Build history of the part. All positions in model axes, mm. Face numbers are marked on the shaded views. A direction names the side the tool comes from. Round coordinates to 2 decimals unless told otherwise and drop trailing zeros. Loops run counter-clockwise (first coordinate to the right, second up) from the corner with the lowest first, then second, coordinate; pieces in that order, holes last.
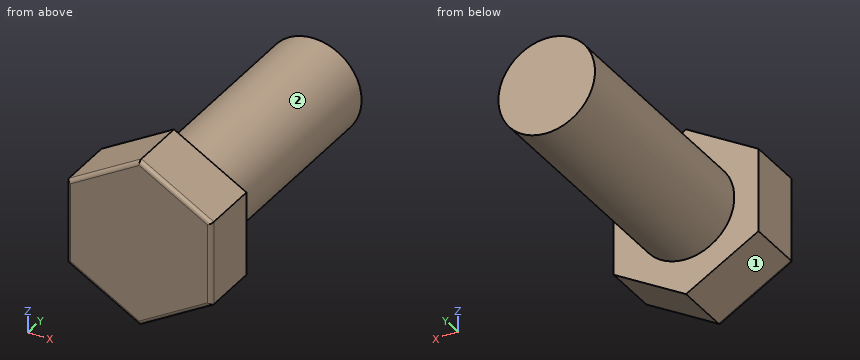
from build123d import *

# Parameters (mm, degrees)
EXTRUDE_1_DEPTH = 15
SKETCH_2_R      = 12
EXTRUDE_2_DEPTH = 60
FILLET_1_R      = 1


with BuildPart() as part:
    # 草圖1 → 填料-伸長1 (new body)
    with BuildSketch(Plane(origin=(0, 0, 0), x_dir=(1, 0, 0), z_dir=(0, 1, 0))):
        Polygon((18, -10.392304845), (18, 10.392304845), (0, 20.784609691), (-18, 10.392304845), (-18, -10.392304845), (0, -20.784609691), align=None)
    extrude(amount=EXTRUDE_1_DEPTH)

    # 草圖2 → 填料-伸長2 (add)
    with BuildSketch(Plane(origin=(0, 15, 0), x_dir=(1, 0, 0), z_dir=(0, 1, 0))):
        Circle(SKETCH_2_R)
    extrude(amount=EXTRUDE_2_DEPTH)

    # 圓角1
    fillet_1_edges = [part.edges().sort_by_distance(p)[0] for p in [
        (18, 0, 0),
        (9, 0, 15.588457268),
        (-9, 0, 15.588457268),
        (-18, 0, 0),
        (-9, 0, -15.588457268),
        (9, 0, -15.588457268),
    ]]
    fillet(fillet_1_edges, radius=FILLET_1_R)


solid = part.part
(1) Pin check, flat tips, straight feed: P1, Ø1, axis at x = 8.5, z = -16, coming from the -Y side; P2, Ø2, axis at y = 30.5, z = -3, coming from the +X side; P3, Ø1, axis at x = 3, y = 10, coming from the +Z side; P4, Ø8, axis at x = -12.5, z = 7, coming from the +Y side. Stop position of each tip, or through.
Responses:
P1: stops at y = 0.2
P2: stops at x = 11.83
P3: stops at z = 19.34
P4: stops at y = 75
(2) Slice it at C-C on z = -7.5. List the corners of the cut face in (x, y).
Responses:
outline: (-18, 1) arc R1 ccw to (-17, 0) - (17, 0) arc R1 ccw to (18, 1) - (18, 15) - (9.37, 15) - (9.37, 75) - (-9.37, 75) - (-9.37, 15) - (-18, 15) - close
(3) Which spindle directions (+Z, -Z, +X, -X, +Y, -Y) get a long thin tool onto all of the face, cutting with end or side? Do the marked faces 1 and 2. Say none if no direction does.
Responses:
face 1: -Z, -X, +Y, -Y
face 2: +Y
(4) Probe line 1 (Y direction, x = -11, z = 9); line 2 (X direction, y = 56, z = -6.5); line 3 (X direction, y = 19.5, z = -11). List the from-to ranges inside material, lowest first.
Responses:
line 1: y = 0 to 15
line 2: x = -10.09 to 10.09
line 3: x = -4.8 to 4.8
(5) Slice it at D-D on y = 66. List the corners of the cut face in (x, z), plus the area to 3 significant figures.
Responses:
outline: circle Ø24 at (0, 0)
area: 452 mm2
(6) Slice it at B-B on z = 0. List the corners of the cut face in (x, y).
Responses:
outline: (-18, 1) arc R1 ccw to (-17, 0) - (17, 0) arc R1 ccw to (18, 1) - (18, 15) - (12, 15) - (12, 75) - (-12, 75) - (-12, 15) - (-18, 15) - close
(7) Slice it at A-A on y = 7. List the corners of the cut face in (x, z), plus the area to 3 significant figures.
Responses:
outline: (-18, -10.39) - (0, -20.78) - (18, -10.39) - (18, 10.39) - (0, 20.78) - (-18, 10.39) - close
area: 1,120 mm2
